```python
from build123d import *

# Parameters (mm, degrees)
F3_W     = 50
F3_H     = 76.046514
F4_DEPTH = 61.9
F5_R     = 11.27
F6_DEPTH = 61.8


with BuildPart() as f1:
    # F0 (on Front) → F1 (revolve)
    with BuildSketch(Plane.XZ):
        Polygon((47.209889, 0), (61.891673, 62.197552), (0, 62.49862), (0, 0), align=None)
    revolve(axis=Axis((0, 0, 31.24931), (0, 0, 1)))

    # F3 (on offset) → F4 (cut)
    with BuildSketch(Plane.YZ.offset(29)):
        with Locations((0, 28.95349)):
            Rectangle(F3_W, F3_H)
    extrude(amount=F4_DEPTH, mode=Mode.SUBTRACT)

    # F5 (on Top) → F6 (join)
    with BuildSketch(Plane.XY):
        with BuildLine():
            Line((-27.737366, 28.822735), (-106.242556, 28.822735))
            Line((-106.242556, 28.822735), (-106.242556, -28.822735))
            Line((-106.242556, -28.822735), (-28.702144, -28.822735))
            ThreePointArc((-28.702144, -28.822735), (-40.032989, 0.197711), (-27.737366, 28.822735))
        make_face()
        with Locations((-81.947307, 0)):
            Circle(F5_R, mode=Mode.SUBTRACT)
    extrude(amount=F6_DEPTH)

    # F7 (on Front) → F8 (revolve, cut)
    with BuildSketch(Plane.XZ):
        Polygon((0, 62.710572), (0, 0), (44.315554, 0), (60.244557, 62.710572), align=None)
    revolve(axis=Axis((0, 0, 31.355286), (0, 0, 1)), mode=Mode.SUBTRACT)


solid = f1.part
```
Verification items for the finished model (mm, model axes). Coordinates: 2 decimals unless noted, no trailing zeros. Order: outer loops, then holes, each group sorted by start corner. A loop starts at its lowest first (then second) coordinate and runs counter-clockwise, first axis right, second up. Notation, with made-up numbers: (77, 17) -> (118, 17) arc R26 ccw to (118, 43) -> close; hole circle Ø11 at (31.5, 77.5). An arc over 180 degrees is marked (long way). Put each result on its own line as item: value. Start each with the question number.
1) Cross-section at A-A (y = 0). Enter the section's corners in (x, z), plus the area to 3 significant figures.
2) Cross-section at C-C (z = 37). Enter the section's corners in (x, y).
3) Release check for a two-part mould opening along Y. For faces 1 (the flat face through (47, 25, 29)), 2 (the flat face through (-80, -28.823, 30)), 3 (the flat face through (-79, 28.823, 30)), 4 (the flat face through (-60, -3, 0)) record: pulls with the +Y half, pulls with the -Y half, needs draft (parallel to the pull), parting line crosses it, or undercut.
4) Cross-section at D-D (z = 22). Enter the section's corners in (x, y).
5) Go/stop test with flat-tipped pins: pin 1 (10 mm diameter, centred on x = 47.5, z = 28.5, fed in from +Y); pin 2 (3 mm diameter, centred on y = -19.5, z = 42, fed in from +X); pin 3 (6 mm diameter, centred on x = -78, z = 34, fed in from +Y). Record where each tip stops, or that it passes through.
6) Material ranges on L1, parallel to Y at x = 17, z = 25; L2, parallel to X at y = 34.5, z = 27; L3, parallel to Y at x = -21.5, z = 33.5, recorded low to high.
7) Cross-section at B-B (x = -76). Enter the section's corners in (y, z).
Geometry check:
1. outline: (-106.24, 0) -> (-93.22, 0) -> (-93.22, 61.8) -> (-106.24, 61.8) -> close; (-70.68, 0) -> (-44.32, 0) -> (-60.12, 62.21) -> (-61.89, 62.2) -> (-61.8, 61.8) -> (-70.68, 61.8) -> close
1. area: 1,950 mm^2
2. outline: (-106.24, -28.82) -> (-47.95, -28.82) arc R55.94 ccw to (50.05, -25) -> (47.54, -25) arc R53.71 cw (long way) to (47.54, 25) -> (50.05, 25) arc R55.94 ccw to (-47.95, 28.82) -> (-106.24, 28.82) -> close; hole circle Ø22.54 at (-81.95, 0)
3. face 1: undercut
3. face 2: pulls with the -Y half
3. face 3: pulls with the +Y half
3. face 4: needs draft
4. outline: (-106.24, -28.82) -> (-43.76, -28.82) arc R52.4 ccw to (46.06, -25) -> (43.19, -25) arc R49.9 cw (long way) to (43.19, 25) -> (46.06, 25) arc R52.4 ccw to (-43.76, 28.82) -> (-106.24, 28.82) -> close; hole circle Ø22.54 at (-81.95, 0)
5. pin 1: stops at y = 33.49
5. pin 2: stops at x = -50.69
5. pin 3: stops at y = 28.82
6. L1: y = -50.32 to -47.73, 47.73 to 50.32
6. L2: x = -41 to -37.8, 37.8 to 41
6. L3: y = -50.75 to -48.25, 48.25 to 50.75
7. outline: (-28.82, 0) -> (-9.57, 0) -> (-9.57, 61.8) -> (-28.82, 61.8) -> close; (9.57, 0) -> (28.82, 0) -> (28.82, 61.8) -> (9.57, 61.8) -> close
